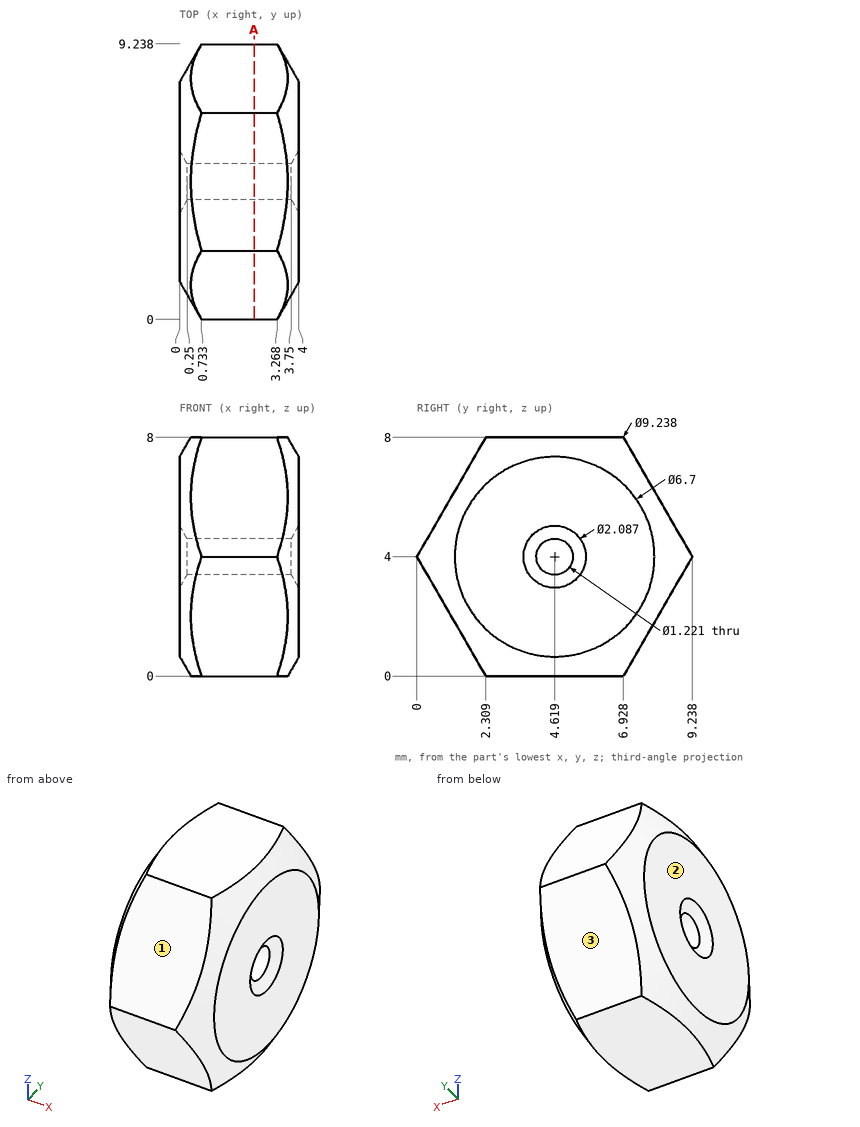
Verification items for this drawing (mm, ordinates from the low corner). Round coordinates to 2 decimals unless told otherwise and drop trailing zeros. Write each loop counter-clockwise with the first axis right and the second up, starting at its lowest first coordinate (ties: lowest second). Pieces come first, ordered by that corner, then holes. Notation, with made-up numbers: (20, 31) - (31, 31) arc R18 cw to (31, 39) - close; hole circle Ø8 at (42, 14). An arc over 180 degrees is marked (long way). One line per item, written item: value.
1. Depth check by flat-ended pin: pin 1 Ø0.7 at (y, z) = (4.62, 4) entering from -X. Enter the tip coordinate at first touch or a pass-through.
The answers:
pin 1: passes through
2. Mould release check, pull along Y, two halves, no side actions. Record for the marked faces 1, 2 and 3: released by +Y, released by -Y, zero draft, split by the parting line, or undercut.
The answers:
face 1: released by -Y
face 2: zero draft
face 3: released by +Y
3. Cross-section at A-A on x = 2.5. Record the boundary of the cut face in (y, z).
The answers:
outline: (0, 4) - (2.31, 0) - (6.93, 0) - (9.24, 4) - (6.93, 8) - (2.31, 8) - close; hole circle Ø1.22 at (4.62, 4)
4. Scan lines: L1, parallel to Y at x = 3.6, z = 2.75 (1 decimal); L2, parallel to Y at x = 0.75, z = 5.25 (1 decimal); L3, parallel to Z at x = 3.15, y = 7.25 (1 decimal). Record each from-to range of solid material in increasing order.
The answers:
L1: y = 0.8 to 8.5
L2: y = 0.7 to 8.5
L3: z = 0.6 to 7.4
